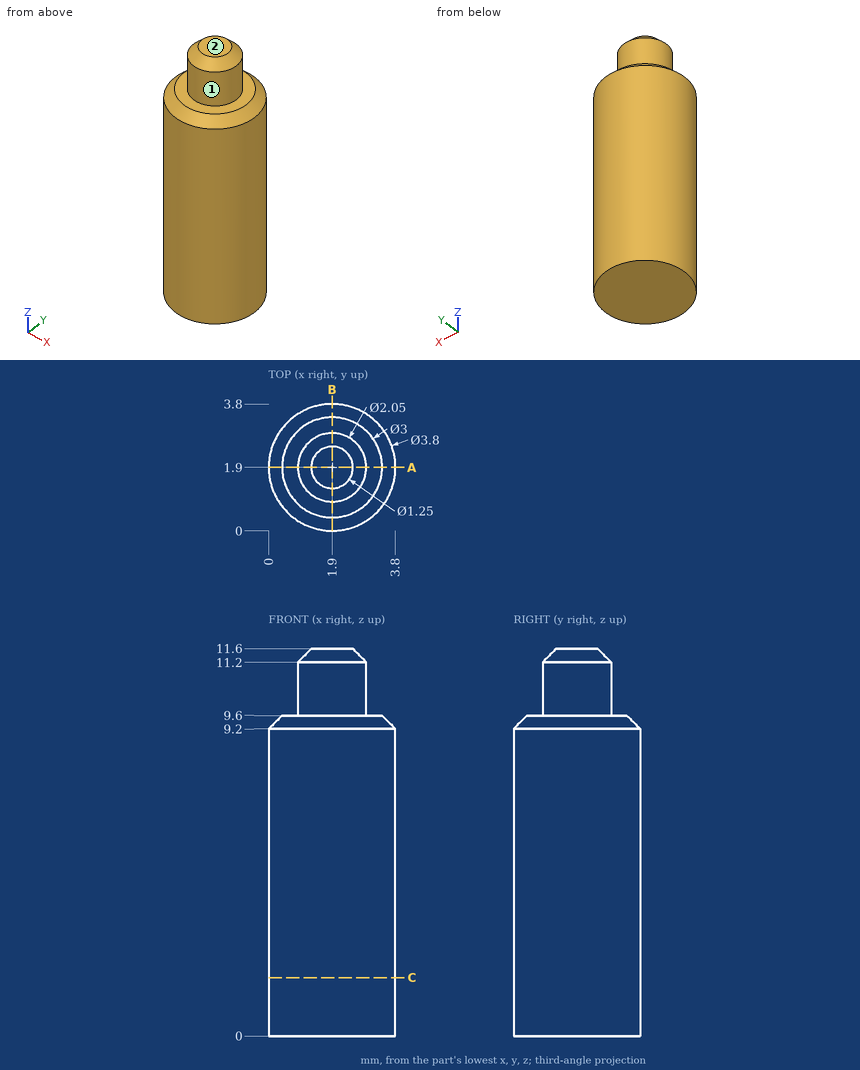
Design review of the part shown in the three views and the two pictorial views. Dimensions are in mm from the part's minimum x, y and z. A direction names the side the tool comes from. Round coordinates to 2 decimals unless told otherwise and drop trailing zeros. Write each loop counter-clockwise with the first axis right and the second up, starting at its lowest first coordinate (ties: lowest second). Pieces come first, ordered by that corner, then holes.
Item 1: For the marked faces 1 and 2, list the 3-axis set-ups (+Z, -Z, +X, -X, +Y, -Y) from which the entire face can be reached by the end or side of a thin tool; tool diameter is ignored.
Item 2: We need section C-C on z = 1.75. Write out the cut boundary in (x, y), and give its area (3 significant figures).
Item 3: We need section A-A on y = 1.9. Write out the cut boundary in (x, z) (3 decimals), and give its area (3 significant figures).
Item 4: For probe 1 along X at (y, z) = (3.5, 6); probe 2 along X at (y, z) = (3.4, 6.25); probe 3 along Y at (x, z) = (1.15, 7.5), list the stretches that pass through material, from the lowest coordinate up.
Item 5: Clearance check with flat-ended pins moving along their axes: pin 1 Ø1 at (x, z) = (2.5, 8.5) entering from +Y; pin 2 Ø1 at (y, z) = (3.5, 2.5) entering from +X. State where each tip first meets the part, or that it passes through.
Returned:
1. face 1: +Z
1. face 2: +Z, +X, -X, +Y, -Y
2. outline: circle Ø3.8 at (1.9, 1.9)
2. area: 11.3 mm2
3. outline: (0, 0) - (3.8, 0) - (3.8, 9.2) - (3.4, 9.6) - (2.925, 9.6) - (2.925, 11.2) - (2.525, 11.6) - (1.275, 11.6) - (0.875, 11.2) - (0.875, 9.6) - (0.4, 9.6) - (0, 9.2) - close
3. area: 40.3 mm2
4. probe 1: x = 0.88 to 2.92
4. probe 2: x = 0.73 to 3.07
4. probe 3: y = 0.15 to 3.65
5. pin 1: stops at y = 3.8
5. pin 2: stops at x = 3.45
